```python
from build123d import *

# Parameters (mm, degrees)
F1_R     = 1.5875
F2_DEPTH = 3.175


with BuildPart() as f2:
    # F1 (on Top) → F2 (new body)
    with BuildSketch(Plane.XY):
        with BuildLine():
            ThreePointArc((-4.0262265136, 5.6513251328), (-5.2977559244, 6.8795791134), (-4.6446774192, 8.5224069649))
            Line((-4.6446774192, 8.5224069649), (-5.3333519733, 9.525))
            Line((-5.3333519733, 9.525), (-34.4962663949, 9.525))
            Line((-34.4962663949, 9.525), (-88.9, 0))
            add(Edge.make_bspline(
                [(-88.9, 0), (-87.2379108001, -1.1763368423), (-77.6465036689, -10.294371312), (-16.7160528872, -9.525), (-13.6749316007, -9.525)],
                knots=[0, 0, 0, 0, 0.3288466474, 1, 1, 1, 1], degree=3))
            Line((-13.6749316007, -9.525), (-2.4758519733, -9.525))
            Line((-2.4758519733, -9.525), (-2.4758519733, -7.5313699697))
            ThreePointArc((-2.4758519733, -7.5313699697), (-4.0325407656, -5.6326204651), (-1.8654348201, -4.4784187937))
            ThreePointArc((-1.8654348201, -4.4784187937), (3.9795795285, -2.7747123701), (3.5571823428, 3.2988688577))
            ThreePointArc((3.5571823428, 3.2988688577), (1.31903069, 3.3310035803), (-0.2092779199, 4.9664326537))
            Line((-0.2092779199, 4.9664326537), (-4.0262265136, 5.6513251328))
        make_face()
        Circle(F1_R, mode=Mode.SUBTRACT)
    extrude(amount=F2_DEPTH)


solid = f2.part
```
CAD build for the part. Positions are in the model's coordinates, mm. A direction names the side the tool comes from. Coordinates: 2 decimals unless noted, no trailing zeros. Use a Markdown table: item, result. Add a question column.
(1) Drill centre lines: line 1 along Y through (x, z) = (0, 1.3); line 2 along X through (y, z) = (-1.25, 2.3); line 3 along Y through (x, z) = (-21.5, 1.3) (3 decimals). Where is each one in solid material? Low to high. Write a range as [from, to].
(2) Flat gauge pins, fed straight in: pin 1 (1.6 mm diameter, centred on y = -9, z = 2, fed in from +X); pin 2 (3.5 mm diameter, centred on x = -2.48, y = -5.94, fed in from -Z); pin 3 (1.5 mm diameter, centred on x = -74, z = 2.5, fed in from +Y). Where does each tip first touch, or does it go through?
(3) Which spindle directions (+Z, -Z, +X, -X, +Y, -Y) get a long thin tool onto all of the face, cutting with end or side? Do faces 4 (the face through (-4.04, -5.67, 1.57)), 5 (the face through (-2.476, -9, 2)). Say none if no direction does.
(4) Pull direction X, two halves, no side cores. Call faces 1 (the face through (1.349, 3.318, 1.565)), 2 (the face through (-32, 0, 3.175)), 3 (the face through (-5.3, 6.9, 1.6)): +X half, -X half, draft (parallel to the pull), parting line (faces both ways), or undercut.
Solved:
| question | item | result |
|---|---|---|
| 1 | line 1 | y = [-4.85, -1.59], [1.59, 4.52] |
| 1 | line 2 | x = [-87.21, -0.98], [0.98, 4.69] |
| 1 | line 3 | y = [-9.546, 9.525] |
| 2 | pin 1 | stops at x = -2.48 |
| 2 | pin 2 | stops at z = 0 |
| 2 | pin 3 | stops at y = 2.74 |
| 3 | face 4 | +Z, -Z |
| 3 | face 5 | +Z, -Z, +X, -Y |
| 4 | face 1 | undercut |
| 4 | face 2 | draft |
| 4 | face 3 | +X half |
